Design review of the part built by this model. Coordinates are the model's own, in mm. Face numbers are marked on the shaded views. A direction names the side the tool comes from. Give positions to 0.01 mm unless a question says otherwise; leave off trailing zeros. Loops run counter-clockwise (first coordinate to the right, second up) from the corner with the lowest first, then second, coordinate; pieces in that order, holes last. Notation, with made-up numbers: M -29.75,86 L 15.25,86 A31 cw 15.25,124 Z; hole C -35,32.5 d10. An arc over 180 degrees is marked long. Use CSV: the item, a comma, the result in double quotes.
from build123d import *

# Parameters (mm, degrees)
F1_DEPTH  = 12.7
F2_R      = 7.112
F3_DEPTH  = 12.701
F4_R      = 12.7
F5_DEPTH  = 4.572
F7_DEPTH  = 12.7
F8_W      = 16.002
F8_H      = 7.874
F9_DEPTH  = 19.05
F10_W     = 16.002
F10_H     = 12.7
F11_DEPTH = 47.752


with BuildPart() as f1:
    # F0 (on Top) → F1 (new body)
    with BuildSketch(Plane.XY):
        Polygon((0, 63.5), (0, 0), (16.002, 0), (16.002, 7.874), (47.498, 7.874), (47.498, 0), (63.5, 0), (63.5, 63.5), (47.498, 63.5), (47.498, 55.626), (16.002, 55.626), (16.002, 63.5), align=None)
    extrude(amount=F1_DEPTH)

    # F2 (on face) → F3 (cut, through all)
    with BuildSketch(Plane.XY.offset(12.7)):
        with Locations((31.75, 31.75)):
            Circle(F2_R)
    extrude(amount=-F3_DEPTH, mode=Mode.SUBTRACT)

    # F4 (on face) → F5 (cut)
    with BuildSketch(Plane.XY.offset(12.7)):
        with Locations((31.75, 31.75)):
            Circle(F4_R)
    extrude(amount=-F5_DEPTH, mode=Mode.SUBTRACT)

    # F6 (on face) → F7 (join)
    with BuildSketch(Plane(origin=(0, 0, 0), x_dir=(0, -1, 0), z_dir=(-1, 0, 0))):
        with BuildLine():
            ThreePointArc((-50.582985, 47.750007), (-59.867423, 43.952356), (-63.5, 34.602097))
            Line((-63.5, 34.602097), (-63.5, 12.7))
            Line((-63.5, 12.7), (0, 12.7))
            Line((0, 12.7), (0, 35.052))
            ThreePointArc((0, 35.052), (-3.71998, 44.032492), (-12.700668, 47.752))
            Line((-12.700668, 47.752), (-50.582985, 47.750007))
        make_face()
        with BuildLine():
            ThreePointArc((-12.7, 42.926), (-4.826, 35.052), (-12.7, 27.178))
            Line((-12.7, 27.178), (-50.807972, 27.178))
            ThreePointArc((-50.807972, 27.178), (-58.681972, 35.052), (-50.807972, 42.926))
            Line((-50.807972, 42.926), (-12.7, 42.926))
        make_face(mode=Mode.SUBTRACT)
    extrude(amount=-F7_DEPTH)

    # F8 (on face) → F9 (join)
    with BuildSketch(Plane(origin=(0, 0, 0), x_dir=(1, 0, 0), z_dir=(0, 0, -1))):
        with Locations((55.499, -3.937)):
            Rectangle(F8_W, F8_H)
        with Locations((55.499, -59.563)):
            Rectangle(F8_W, F8_H)
    extrude(amount=F9_DEPTH)

    # F10 (on face) → F11 (join, through all)
    with BuildSketch(Plane(origin=(0, 7.874, 0), x_dir=(-1, 0, 0), z_dir=(0, 1, 0))):
        with Locations((-55.499, -6.35)):
            Rectangle(F10_W, F10_H)
    extrude(amount=F11_DEPTH)


solid = f1.part
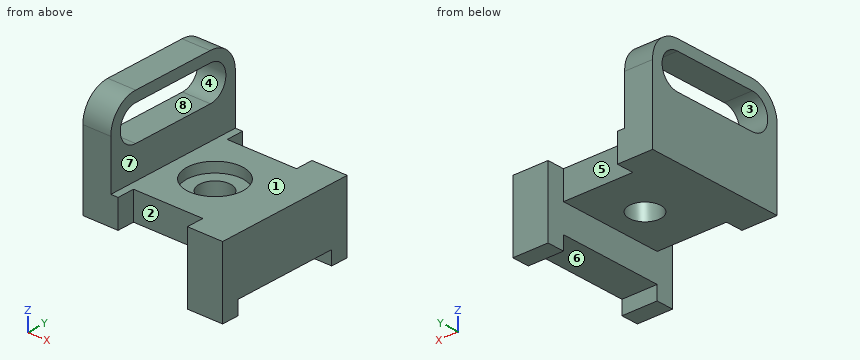
(1) We need section B-B on z = 7. State the section outline as (x, y) points.
A:
outline,"M 0,0 L 16,0 L 16,7.87 L 47.5,7.87 L 47.5,0 L 63.5,0 L 63.5,63.5 L 47.5,63.5 L 47.5,55.63 L 16,55.63 L 16,63.5 L 0,63.5 Z; hole C 31.75,31.75 d14.22"
(2) We need section D-D on z = 33.5. State the section outline as (x, y) points.
A:
outline,"M 0,0 L 12.7,0 L 12.7,4.98 L 0,4.98 Z; M 0,58.53 L 12.7,58.53 L 12.7,63.5 L 0,63.5 Z"
(3) We need section A-A on x = 31.75. State the section outline as (y, z) points.
A:
outline,"M 7.87,0 L 24.64,0 L 24.64,8.13 L 19.05,8.13 L 19.05,12.7 L 7.87,12.7 Z; M 38.86,0 L 55.63,0 L 55.63,12.7 L 44.45,12.7 L 44.45,8.13 L 38.86,8.13 Z"
(4) Clearance check with flat-ended pins moving along their axes: P1, Ø5, axis at x = 16, y = 9, coming from the -Z side; P2, Ø12, axis at x = 25.5, y = 35.5, coming from the +Z side; P3, Ø13, axis at x = 9, z = 18, coming from the +Y side. State where each tip first meets the part, or that it passes through.
A:
P1,"z = 0"
P2,"z = 12.7"
P3,"y = 63.5"
(5) The part is to be moulded in two halves that separate along Z. For the marked faces 1, 2, 3 and 4, say which applies: released by +Z, released by -Z, zero draft, split by the parting line, or undercut.
A:
face 1,"released by +Z"
face 2,"zero draft"
face 3,"undercut"
face 4,"undercut"
(6) We need section C-C on y = 57. State the section outline as (x, z) points.
A:
outline,"M 0,0 L 16,0 L 16,12.7 L 12.7,12.7 L 12.7,30.19 L 0,30.19 Z; M 0,39.92 L 12.7,39.92 L 12.7,46.14 L 0,46.14 Z; M 47.5,-19.05 L 63.5,-19.05 L 63.5,12.7 L 47.5,12.7 Z"
(7) Wall thickness on line 1 along Y through (x, z) = (31.75, 3.5); line 2 along Z through (x, y) = (11, 24.5); line 3 along Y through (x, z) = (31.75, 9.7): over which ranges is each line inside the solid? List them lowest first. Write a range as [from, to].
A:
line 1,"[7.87, 24.64], [38.86, 55.63]"
line 2,"[0, 27.18], [42.93, 47.75]"
line 3,"[7.87, 19.05], [44.45, 55.63]"
(8) Machinability: for the marked faces 5, 6, 7 and 8, which of the approach directions +Z, -Z, +X, -X, +Y, -Y give a long, thin tool a straight path to every point of the face, cutting with its end or side? Answer none if there is none.
A:
face 5,"+Z, -Z, +Y"
face 6,"-Z, +X, -X"
face 7,"+Z, +X, +Y, -Y"
face 8,"+X, -X"
